Autodesk Inventor part; units mm, degrees
ref_plane "YZ Plane" through (0, 0, 0) normal (1, 0, 0) x (0, 1, 0)
ref_plane "XZ Plane" through (0, 0, 0) normal (0, 1, 0) x (-1, 0, 0)
ref_plane "XY Plane" through (0, 0, 0) normal (0, 0, 1) x (1, 0, 0)
sketch "Boceto1" plane through (0, 0, 0) normal (0, 1, 0) x (-1, 0, 0)
  line L0 (-5.4361, 12.1513) -> (1.0639, 12.1513)
  line L1 (1.0639, 12.1513) -> (1.0639, -17.8487)
  line L2 (1.0639, -17.8487) -> (-5.4361, -17.8487)
  line L3 (-5.4361, -17.8487) -> (-5.4361, -18.8487)
  line L4 (-5.4361, -18.8487) -> (2.0639, -18.8487)
  line L5 (2.0639, -18.8487) -> (2.0639, 13.1513)
  line L6 (2.0639, 13.1513) -> (-5.4361, 13.1513)
  line L7 (-5.4361, 13.1513) -> (-5.4361, 12.1513)
  point P0 (0, 0)
  point P1 (0, 0)
  dimension "d0" = 6.5
  dimension "d1" = 30
  dimension "d2" = 1
  dimension "d3" = 7.5
  dimension "d4" = 32
extrude "Extrusión1" add sketch "Boceto1" along normal blind 340
properties part number "Tapa cable canal 340mm"
Read the model definition and answer for the solid it produces. Units are mm, in the model's axes. A direction names the side the tool comes from. Round coordinates to 2 decimals unless told otherwise and drop trailing zeros. Order: outer loops, then holes, each group sorted by start corner. A loop starts at its lowest first (then second) coordinate and runs counter-clockwise, first axis right, second up.
1) The part is cut by section B-B on y = 133.5. Write down the section's boundary in (x, z), plus the area to 3 significant figures.
2) The part is cut by section C-C on z = -3. Write down the section's boundary in (x, y), plus the area to 3 significant figures.
3) Flat-ended cylindrical pins translate along their axes: pin 1 (10 mm diameter, centred on y = 79, z = -15, fed in from +X); pin 2 (2 mm diameter, centred on y = 144, z = -9, fed in from +X). Find the tip coordinate at first contact, or state that the pin passes through.
4) The mould has two halves that part along Z. Classify faces 1 (the face through (-2.064, 168, -3)), 2 (the face through (2, 168, -18.849)), 3 (the face through (-1.064, 168, -3)): released by +Z, released by -Z, zero draft, split by the parting line, or undercut.
5) The part is cut by section A-A on x = 2.75. Write down the section's boundary in (y, z).
6) Straight lines are drawn through the part: L1, parallel to Z at x = -0.25, y = 113; L2, parallel to X at y = 220, z = 7.5. For each, find the intervals that lie inside material, in ascending order.
7) For faces 4 (the face through (2, 168, 12.151)), 5 (the face through (2, 168, 13.151)), determine the directions among +Z, -Z, +X, -X, +Y, -Y from which every point of the face is accessible in a straight line to the end or side of a thin tool.
Resolved:
1. outline: (-2.06, -18.85) - (5.44, -18.85) - (5.44, -17.85) - (-1.06, -17.85) - (-1.06, 12.15) - (5.44, 12.15) - (5.44, 13.15) - (-2.06, 13.15) - close
1. area: 45.0 mm2
2. outline: (-2.06, 0) - (-1.06, 0) - (-1.06, 340) - (-2.06, 340) - close
2. area: 340 mm2
3. pin 1: stops at x = 5.44
3. pin 2: stops at x = -1.06
4. face 1: zero draft
4. face 2: released by -Z
4. face 3: undercut
5. outline: (0, -18.85) - (340, -18.85) - (340, -17.85) - (0, -17.85) - close; (0, 12.15) - (340, 12.15) - (340, 13.15) - (0, 13.15) - close
6. L1: z = -18.85 to -17.85, 12.15 to 13.15
6. L2: x = -2.06 to -1.06
7. face 4: +X, +Y, -Y
7. face 5: +Z, +X, -X, +Y, -Y
